from build123d import *

# Parameters (mm, degrees)
CYLINDER_R       = 2
CYLINDER_DEPTH   = 100
ARRAY002_X_COUNT = 2
ARRAY002_X_PITCH = 77
BOX009_W         = 30
BOX009_H         = 36
BOX009_DEPTH     = 20
BOX001_W         = 143.4
BOX001_H         = 71
BOX001_DEPTH     = 17.3
BOX_W            = 147.4
BOX_H            = 74
BOX_DEPTH        = 16.8
FILLET_R         = 1.5


with BuildPart() as obj1:
    # Cylinder → Cylinder (new body)
    with BuildSketch(Plane(origin=(9.5, -16, 3.5), x_dir=(1, 0, 0), z_dir=(0, 1, 0))):
        Circle(CYLINDER_R)
    extrude(amount=CYLINDER_DEPTH)

    # Array002 X: obj1_2


with BuildPart() as obj1_1:
    add(obj1.part)
    with Locations(*[(i * ARRAY002_X_PITCH, 0, 0) for i in range(1, ARRAY002_X_COUNT)]):
        add(obj1.part)


with BuildPart() as obj1_2:
    # Body placement: moved
    add(obj1_1.part.moved(Location((2.2, 0, 2.9))))


with BuildPart() as usb_extent_hole:
    # Box009 → Box009 (new body)
    with BuildSketch(Plane(origin=(131, 13, 1.4), x_dir=(1, 0, 0), z_dir=(0, 0, 1))):
        with Locations((15, 18)):
            Rectangle(BOX009_W, BOX009_H)
    extrude(amount=BOX009_DEPTH)


with BuildPart() as bottom_body_hole_fusion:
    # Box001 → Box001 (new body)
    with BuildSketch(Plane(origin=(2, 1.5, 1), x_dir=(1, 0, 0), z_dir=(0, 0, 1))):
        with Locations((71.7, 35.5)):
            Rectangle(BOX001_W, BOX001_H)
    extrude(amount=BOX001_DEPTH)

    # Fusion: union obj1, usb extent hole
    add(obj1_2.part)
    add(usb_extent_hole.part)


with BuildPart() as bottom_fillet:
    # Box → Box (new body)
    with BuildSketch(Plane.XY):
        with Locations((73.7, 37)):
            Rectangle(BOX_W, BOX_H)
    extrude(amount=BOX_DEPTH)

    # Cut: cut bottom body hole fusion
    add(bottom_body_hole_fusion.part, mode=Mode.SUBTRACT)

    # Fillet
    fillet_edges = [bottom_fillet.edges().sort_by_distance(p)[0] for p in [
        (0, 0, 8.4),
        (0, 74, 8.4),
        (147.4, 0, 8.4),
        (147.4, 74, 8.4),
        (145.4, 72.5, 8.9),
        (145.4, 1.5, 8.9),
        (2, 72.5, 8.9),
        (2, 1.5, 8.9),
    ]]
    fillet(fillet_edges, radius=FILLET_R)


solid = bottom_fillet.part
Geometry check sheet. Reference: the model listing, model coordinates, mm. A direction names the side the tool comes from. Give positions to 0.01 mm unless a question says otherwise; leave off trailing zeros. Order: outer loops, then holes, each group sorted by start corner. A loop starts at its lowest first (then second) coordinate and runs counter-clockwise, first axis right, second up. Notation, with made-up numbers: (77.25, -11.5) - (110.25, -11.5) arc R15 cw to (110.25, 14.5) - close; hole circle Ø3 at (47, 76.5). An arc over 180 degrees is marked (long way). Use one line per item in the form item = value.
1) Depth check by flat-ended pin: pin 1 Ø1.6 at (x, y) = (147, 30.5) entering from +Z; pin 2 Ø3 at (x, z) = (11.7, 6.4) entering from -Y; pin 3 Ø2 at (x, y) = (55, 12) entering from +Z; pin 4 Ø4.5 at (y, z) = (21, 7.5) entering from +X. Enter the tip coordinate at first touch or a pass-through.
Working result:
pin_1 = 1.4
pin_2 = through
pin_3 = 1
pin_4 = 2
2) Sectioned sample at A-A (x = 88.7). Record the boundary of the cut face in (y, z).
Working result:
outline = (0, 0) - (74, 0) - (74, 4.4) - (72.5, 4.4) - (72.5, 1) - (1.5, 1) - (1.5, 4.4) - (0, 4.4) - close; (0, 8.4) - (1.5, 8.4) - (1.5, 16.8) - (0, 16.8) - close; (72.5, 8.4) - (74, 8.4) - (74, 16.8) - (72.5, 16.8) - close
3) Sectioned sample at C-C (x = 110). Record the boundary of the cut face in (y, z), and give its area (3 significant figures).
Working result:
outline = (0, 0) - (74, 0) - (74, 16.8) - (72.5, 16.8) - (72.5, 1) - (1.5, 1) - (1.5, 16.8) - (0, 16.8) - close
area = 121 mm^2
4) Material ranges on probe 1 along X at (y, z) = (10, 5.25); probe 2 along Y at (x, z) = (105.5, 8.5); probe 3 along Z at (x, y) = (88.7, 73.5), recorded low to high. Write a range as from..to.
Working result:
probe_1 = 0..2, 145.4..147.4
probe_2 = 0..1.5, 72.5..74
probe_3 = 0..4.4, 8.4..16.8
5) Sectioned sample at D-D (z = 6.4). Count the separate pieces of the cut face and the enclosed holes in it, and give its area (3 significant figures).
Working result:
separate_pieces = 5
enclosed_holes = 0
area = 630 mm^2
6) Access from +Z, -Z, +X, -X, +Y, -Y to the whole of each face (thin tool, end or side, straight path). Record for faces 4 (the face through (2, 37, 9)), 5 (the face through (89.623, 73.24, 8.174)).
Working result:
face_4 = +Z
face_5 = +Y, -Y
7) Draft check along Y on faces 1 (the face through (145.4, 52, 9)), 2 (the face through (73, 38, 0)), 3 (the face through (73, 0, 8)). Enter one of: released by +Y, released by -Y, zero draft, split by the parting line, or undercut.
Working result:
face_1 = undercut
face_2 = zero draft
face_3 = released by -Y
8) Sectioned sample at B-B (y = 30). Record the boundary of the cut face in (x, z).
Working result:
outline = (0, 0) - (147.4, 0) - (147.4, 1.4) - (145.4, 1.4) - (145.4, 1) - (2, 1) - (2, 16.8) - (0, 16.8) - close
